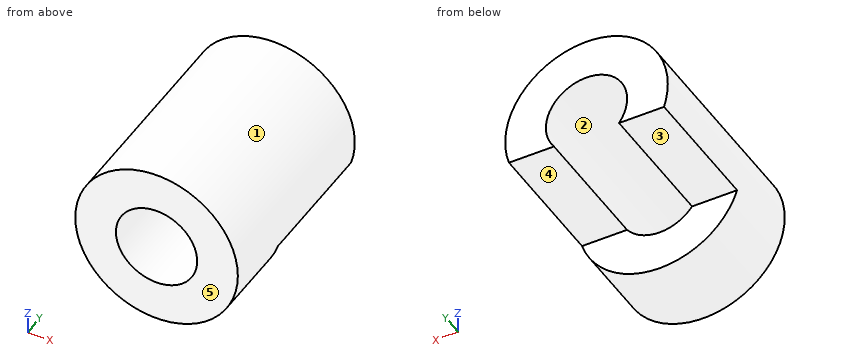
Autodesk Inventor part; units mm, degrees
ref_plane "YZ Plane" through (0, 0, 0) normal (1, 0, 0) x (0, 1, 0)
ref_plane "XZ Plane" through (0, 0, 0) normal (0, 1, 0) x (-1, 0, 0)
ref_plane "XY Plane" through (0, 0, 0) normal (0, 0, 1) x (1, 0, 0)
sketch "Sketch1" plane through (0, 0, 0) normal (0, 1, 0) x (-1, 0, 0)
  circle A0 centre (0, 0) radius 1.5875
  circle A1 centre (0, 0) radius 3.175
  dimension "d0" = 3.175
  dimension "d1" = 6.35
extrude "Extrusion1" add sketch "Sketch1" along normal blind 8.128
sketch "Sketch2" plane through (0, 8.128, 0) normal (0, 1, 0) x (1, 0, 0)
  line L0 (-3.175, 3.7564) -> (3.175, 3.7564)
  line L1 (3.175, 3.7564) -> (3.175, 0.9525)
  line L2 (3.175, 0.9525) -> (-3.175, 0.9525)
  line L3 (-3.175, 0.9525) -> (-3.175, 3.7564)
  point P0 (0, 0)
  dimension "d4" = 3.175
  dimension "d5" = 6.35
  dimension "d6" = 0.9525
extrude "Extrusion2" cut sketch "Sketch2" against normal blind 5.08
properties part number "ShaftCollar" material "Brass, Soft Yellow"
Model file for the job. Use its own axes, mm. Face numbers are marked on the shaded views. A direction names the side the tool comes from. Give positions to 0.01 mm unless a question says otherwise; leave off trailing zeros. Loops run counter-clockwise (first coordinate to the right, second up) from the corner with the lowest first, then second, coordinate; pieces in that order, holes last. Notation, with made-up numbers: (-4, -19) - (35, -19) arc R27 ccw to (35, 1) - close; hole circle Ø10 at (73.25, 25.25). An arc over 180 degrees is marked (long way). One line per item, written item: value. Start each with the question number.
1. Pull direction X, two halves, no side cores. Call the marked faces 1, 2 and 3: pulls with the +X half, pulls with the -X half, needs draft (parallel to the pull), parting line crosses it, or undercut.
2. Which spindle directions (+Z, -Z, +X, -X, +Y, -Y) get a long thin tool onto all of the face, cutting with end or side? Do the marked faces 4 and 5. Say none if no direction does.
3. Slice it at A-A (z = 0). List the corners of the cut face in (x, y) (1 decimal).
4. Slice it at D-D (x = -2.5). List the corners of the cut face in (y, z).
5. Probe L1, parallel to X at y = 3.5, z = 0 (1 decimal); L2, parallel to Y at x = -1, z = -1.5. List the from-to ranges inside material, lowest first. Write a range as from..to.
6. Pin check, flat tips, straight feed: pin 1 (1.4 mm diameter, centred on x = 2, y = 6, fed in from -Z); pin 2 (2 mm diameter, centred on y = 2.5, z = -1, fed in from +X) (3 decimals); pin 3 (2 mm diameter, centred on y = 2.5, z = 2, fed in from -X); pin 4 (1.8 mm diameter, centred on x = 1.5, z = -2, fed in from +Y). Stop position of each tip, or through.
7. Slice it at B-B (x = 0). List the corners of the cut face in (y, z) (1 decimal).
Solution:
1. face 1: parting line crosses it
1. face 2: undercut
1. face 3: needs draft
2. face 4: -Z, +X, -X, +Y
2. face 5: +Z, -Z, +X, -X, -Y
3. outline: (-3.2, 0) - (-1.6, 0) - (-1.6, 8.1) - (-3.2, 8.1) - close; (1.6, 0) - (3.2, 0) - (3.2, 8.1) - (1.6, 8.1) - close
4. outline: (0, -1.96) - (3.05, -1.96) - (3.05, -0.95) - (8.13, -0.95) - (8.13, 1.96) - (0, 1.96) - close
5. L1: x = -3.2..-1.6, 1.6..3.2
5. L2: y = 0..3.05
6. pin 1: stops at z = -0.95
6. pin 2: stops at x = 3.175
6. pin 3: stops at x = -3.01
6. pin 4: stops at y = 3.05
7. outline: (0, -3.2) - (3, -3.2) - (3, -1.6) - (0, -1.6) - close; (0, 1.6) - (8.1, 1.6) - (8.1, 3.2) - (0, 3.2) - close
